Can you work these out from the model? Positions are in its coordinate system, mm. A direction names the side the tool comes from. Coordinates: 2 decimals unless noted, no trailing zeros. Order: outer loops, then holes, each group sorted by start corner. A loop starts at its lowest first (then second) coordinate and runs counter-clockwise, first axis right, second up.
```python
from build123d import *

# Parameters (mm, degrees)
EXTRUDE_1_DEPTH                  = 5.8
SKETCH_2_W                       = 2.5
SKETCH_2_H                       = 1
EXTRUDE_2_DEPTH                  = 8.2
SKETCH_3_W                       = 2.5
SKETCH_3_H                       = 2
EXTRUDE_3_DEPTH                  = 0.2
CHAMFER_1_SIZE                   = 0.2
FILLET_1_R                       = 1
SKETCH_4_W                       = 1
SKETCH_4_H                       = 1
CUT_EXTRUDE_1_DEPTH              = 0.5
CUT_EXTRUDE_1_DRAFT              = -44
PATTERN_LINEAR_1_COPY_1_SKETCH_W = 1
PATTERN_LINEAR_1_COPY_1_SKETCH_H = 1
PATTERN_LINEAR_1_COPY_1_DEPTH    = 0.5
PATTERN_LINEAR_1_COPY_1_DRAFT    = -44


with BuildPart() as part:
    # Эскиз1 → Бобышка-Вытянуть1 (new body)
    with BuildSketch(Plane.XY):
        Polygon((0, 0), (0, 3.2), (5, 3.2), (5, 0), (4.2, 0), (4.2, 1.2), (3.2, 1.2), (3.2, 0), (1.8, 0), (1.8, 1.2), (0.8, 1.2), (0.8, 0), align=None)
    extrude(amount=EXTRUDE_1_DEPTH)

    # Эскиз2 → Бобышка-Вытянуть2 (add)
    with BuildSketch(Plane(origin=(0, 3.2, 0), x_dir=(1, 0, 0), z_dir=(0, 1, 0))):
        with Locations((2.5, -0.5)):
            Rectangle(SKETCH_2_W, SKETCH_2_H)
    extrude(amount=EXTRUDE_2_DEPTH)

    # Эскиз3 → Бобышка-Вытянуть3 (add)
    with BuildSketch(Plane.XY.offset(1)):
        with Locations((2.5, 6.6)):
            Rectangle(SKETCH_3_W, SKETCH_3_H)
    extrude(amount=EXTRUDE_3_DEPTH)

    # Фаска1
    chamfer_1_edges = [part.edges().sort_by_distance(p)[0] for p in [
        (2.5, 5.6, 1.2),
        (2.5, 7.6, 1.2),
    ]]
    chamfer(chamfer_1_edges, length=CHAMFER_1_SIZE - 0.0001)  # a hair under: the kernel refuses the full size

    # Скругление1
    fillet_1_edges = [part.edges().sort_by_distance(p)[0] for p in [
        (1.25, 11.4, 0.5),
        (3.75, 11.4, 0.5),
    ]]
    fillet(fillet_1_edges, radius=FILLET_1_R)


with BuildPart() as cut_extrude_1_tool:
    # Эскиз4 → Вырез-Вытянуть1 (with draft: the straight prism first)
    with BuildSketch(Plane(origin=(0, 3.2, 0), x_dir=(1, 0, 0), z_dir=(0, 1, 0))):
        with Locations((1.25, -2.6)):
            Rectangle(SKETCH_4_W, SKETCH_4_H)
    extrude(amount=-CUT_EXTRUDE_1_DEPTH)
    # Вырез-Вытянуть1: the draft: its side faces are tilted about the plane it starts from
    cut_extrude_1_sides = [cut_extrude_1_tool.faces().sort_by_distance(p)[0] for p in [
        (0.75, 2.95, 2.6),
        (1.25, 2.95, 3.1),
        (1.75, 2.95, 2.6),
        (1.25, 2.95, 2.1),
    ]]
    draft(cut_extrude_1_sides, Plane(origin=(0, 3.2, 0), x_dir=(1, 0, 0), z_dir=(0, 1, 0)), CUT_EXTRUDE_1_DRAFT)


with BuildPart() as part_1:
    add(part.part)

    # Вырез-Вытянуть1: cut by cut_extrude_1_tool
    add(cut_extrude_1_tool.part, mode=Mode.SUBTRACT)


with BuildPart() as pattern_linear_1_copy_1_tool:
    # Линейный массив1 copy 1 sketch → Линейный массив1 copy 1 (with draft: the straight prism first)
    with BuildSketch(Plane(origin=(2.54, 3.2, 0), x_dir=(1, 0, 0), z_dir=(0, 1, 0))):
        with Locations((1.25, -2.6)):
            Rectangle(PATTERN_LINEAR_1_COPY_1_SKETCH_W, PATTERN_LINEAR_1_COPY_1_SKETCH_H)
    extrude(amount=-PATTERN_LINEAR_1_COPY_1_DEPTH)
    # Линейный массив1 copy 1: the draft: its side faces are tilted about the plane it starts from
    pattern_linear_1_copy_1_sides = [pattern_linear_1_copy_1_tool.faces().sort_by_distance(p)[0] for p in [
        (3.29, 2.95, 2.6),
        (3.79, 2.95, 3.1),
        (4.29, 2.95, 2.6),
        (3.79, 2.95, 2.1),
    ]]
    draft(pattern_linear_1_copy_1_sides, Plane(origin=(2.54, 3.2, 0), x_dir=(1, 0, 0), z_dir=(0, 1, 0)), PATTERN_LINEAR_1_COPY_1_DRAFT)


with BuildPart() as part_2:
    add(part_1.part)

    # Линейный массив1 copy 1: cut by pattern_linear_1_copy_1_tool
    add(pattern_linear_1_copy_1_tool.part, mode=Mode.SUBTRACT)


solid = part_2.part
```
1. Imagine slicing it at D-D on y = 10. Please give me the cut outline in (x, z), then the cut area to 3 significant figures.
Completed:
outline: (1.25, 0) - (3.75, 0) - (3.75, 1) - (1.25, 1) - close
area: 2.50 mm2
2. Thinking about a two-plate mould opening in X: for faces 1 (the flat face through (1, 1.2, 3)), 2 (the flat face through (3, 0, 3)), 3 (the flat face through (1.25, 6.7, 0.5)), 4 (the flat face through (3.2, 1, 3)), which applies, pulls with the +X half, pulls with the -X half, needs draft (parallel to the pull), parting line crosses it, or undercut?
Completed:
face 1: undercut
face 2: needs draft
face 3: pulls with the -X half
face 4: undercut
3. Imagine slicing it at B-B on x = 4.75. Please give me the cut outline in (y, z).
Completed:
outline: (0, 0) - (3.2, 0) - (3.2, 5.8) - (0, 5.8) - close
4. Imagine slicing it at A-A on z = 0.45. Please give me the cut outline in (x, y).
Completed:
outline: (0, 0) - (0.8, 0) - (0.8, 1.2) - (1.8, 1.2) - (1.8, 0) - (3.2, 0) - (3.2, 1.2) - (4.2, 1.2) - (4.2, 0) - (5, 0) - (5, 3.2) - (3.75, 3.2) - (3.75, 10.4) arc R1 ccw to (2.75, 11.4) - (2.25, 11.4) arc R1 ccw to (1.25, 10.4) - (1.25, 3.2) - (0, 3.2) - close
5. On a 3-axis mill with a long thin cutter (end or side, diameter ignored), from which of +Z, -Z, +X, -X, +Y, -Y can I reach the whole of each face in a straight line? I mean faces 5 (the flat face through (3.75, 6.7, 0.5)), 6 (the flat face through (2, 4, 1)), 7 (the flat face through (5, 2, 3)), 8 (the flat face through (0.8, 1, 3)), 9 (the flat face through (2, 9, 1)). Say none if no direction works.
Completed:
face 5: +Z, -Z, +X, +Y
face 6: +Z, +X, -X
face 7: +Z, -Z, +X, +Y, -Y
face 8: +Z, -Z, -Y
face 9: +Z, +X, -X, +Y
6. I'm going to push flat-ended pins straight in: pin 1 (0.8 mm diameter, centred on x = 2.5, y = 6.5, fed in from +Z); pin 2 (1.5 mm diameter, centred on y = 4.5, z = 2, fed in from +X); pin 3 (0.7 mm diameter, centred on x = 3, y = 4.5, fed in from +Z); pin 4 (1.3 mm diameter, centred on y = 6.5, z = 0.5, fed in from +X). Where does each tip first touch, or does it pass through?
Completed:
pin 1: stops at z = 1.2
pin 2: passes through
pin 3: stops at z = 1
pin 4: stops at x = 3.75
7. Please list where these lines run through material, in increasing order: probe 1 along X at (y, z) = (1, 5.3); probe 2 along X at (y, z) = (8.5, 0.8); probe 3 along Y at (x, z) = (2.95, 2.9).
Completed:
probe 1: x = 0 to 0.8, 1.8 to 3.2, 4.2 to 5
probe 2: x = 1.25 to 3.75
probe 3: y = 0 to 3.2
8. Imagine slicing it at C-C on z = 5.25. Please give me the cut outline in (x, y).
Completed:
outline: (0, 0) - (0.8, 0) - (0.8, 1.2) - (1.8, 1.2) - (1.8, 0) - (3.2, 0) - (3.2, 1.2) - (4.2, 1.2) - (4.2, 0) - (5, 0) - (5, 3.2) - (0, 3.2) - close
